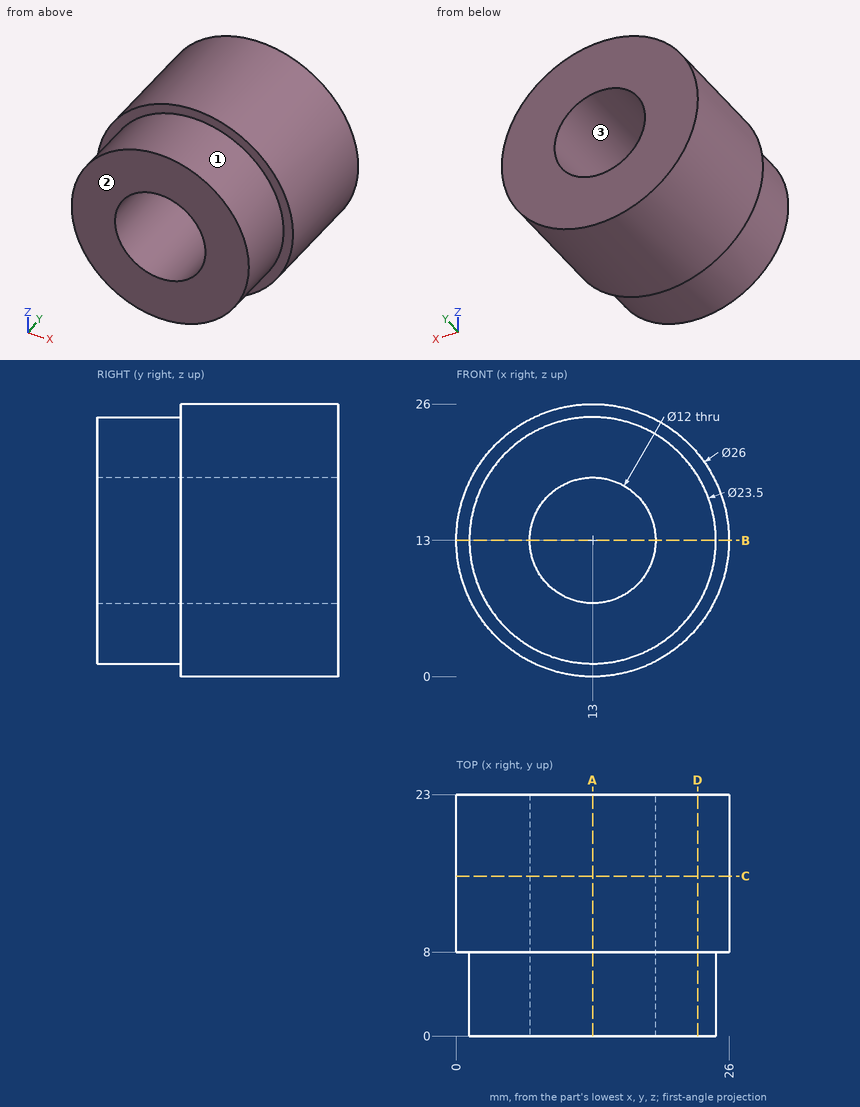
Print and shaded views of the part. All mm, measured from the part's lowest x, y and z. Round coordinates to 2 decimals unless told otherwise and drop trailing zeros. Write each loop counter-clockwise with the first axis right and the second up, starting at its lowest first coordinate (ties: lowest second). Pieces come first, ordered by that corner, then holes. Notation, with made-up numbers: (82.25, 33.5) -> (103.25, 33.5) arc R16 ccw to (103.25, 44.5) -> close; hole circle Ø4 at (-25.5, 11). An arc over 180 degrees is marked (long way). Answer in a Markdown table with one row per item. Add a question column.
Item 1: Mould opens along X. For the marked faces 1, 2 and 3 say: pulls with the +X half, pulls with the -X half, needs draft (parallel to the pull), parting line crosses it, or undercut.
Item 2: Drill centre lines: line 1 (Z direction, x = 13, y = 11.5); line 2 (Y direction, x = 23.25, z = 6.75); line 3 (X direction, y = 7, z = 17). Where is each one in solid material? Low to high. Write a range as from..to.
Item 3: Saw through at C-C, the plane y = 15.25. Write the cut outline in (x, z), then the cut area to 3 significant figures.
Item 4: Saw through at D-D, the plane x = 23. Write the cut outline in (y, z).
Item 5: Saw through at A-A, the plane x = 13. Write the cut outline in (y, z), then the cut area to 3 significant figures.
Item 6: Saw through at B-B, the plane z = 13. Write the cut outline in (x, y).
Item 7: Drop flat-ended pins along their axis: pin 1 Ø4 at (y, z) = (17, 23) entering from +X; pin 2 Ø8 at (x, z) = (16, 18.5) entering from -Y; pin 3 Ø2 at (y, z) = (3, 7.5) entering from +X; pin 4 Ø1.5 at (y, z) = (12, 18.5) entering from -X. Give the stop position or say it passes through.
Findings below:
| question | item | result |
|---|---|---|
| 1 | face 1 | parting line crosses it |
| 1 | face 2 | needs draft |
| 1 | face 3 | undercut |
| 2 | line 1 | z = 0..7, 19..26 |
| 2 | line 2 | y = 8..23 |
| 2 | line 3 | x = 1.95..8.53, 17.47..24.05 |
| 3 | outline | circle Ø26 at (13, 13); hole circle Ø12 at (13, 13) |
| 3 | area | 418 mm^2 |
| 4 | outline | (0, 6.83) -> (8, 6.83) -> (8, 4.69) -> (23, 4.69) -> (23, 21.31) -> (8, 21.31) -> (8, 19.17) -> (0, 19.17) -> close |
| 5 | outline | (0, 1.25) -> (8, 1.25) -> (8, 0) -> (23, 0) -> (23, 7) -> (0, 7) -> close; (0, 19) -> (23, 19) -> (23, 26) -> (8, 26) -> (8, 24.75) -> (0, 24.75) -> close |
| 5 | area | 302 mm^2 |
| 6 | outline | (0, 8) -> (1.25, 8) -> (1.25, 0) -> (7, 0) -> (7, 23) -> (0, 23) -> close; (19, 0) -> (24.75, 0) -> (24.75, 8) -> (26, 8) -> (26, 23) -> (19, 23) -> close |
| 7 | pin 1 | stops at x = 23.25 |
| 7 | pin 2 | stops at y = 0 |
| 7 | pin 3 | stops at x = 23.85 |
| 7 | pin 4 | stops at x = 0.9 |
